from build123d import *

# Parameters (mm, degrees)
F0_W          = 457.2
F0_H          = 368.3
F1_DEPTH      = 6.35
F2_W          = 19.05
F2_H          = 330.2
F2_W_2        = 177.8
F2_H_2        = 19.05
F3_DEPTH      = 63.5
F4_W          = 203.2
F4_H          = 38.1
F4_W_2        = 374.65
F5_DEPTH      = 19.05
F8_DEPTH      = 125.9670187868
F8_DEPTH_BACK = 65.6385295619


# Not quite as in the source:
# - a feature names something its author has since deleted; it is built from what else it names


with BuildPart() as f1:
    # F0 (on Top) → F1 (new body)
    with BuildSketch(Plane.XY):
        with Locations((228.6, 184.15)):
            Rectangle(F0_W, F0_H)
    extrude(amount=F1_DEPTH)

    # F2 (on face) → F3 (join)
    with BuildSketch(Plane.XY.offset(6.35)):
        with Locations((9.525, 184.15)):
            Rectangle(F2_W, F2_H)
        Polygon((0, 368.3), (0, 349.25), (19.05, 349.25), (457.2, 349.25), (457.2, 368.3), align=None)
        Polygon((0, 19.05), (0, 0), (457.2, 0), (457.2, 19.05), (19.05, 19.05), align=None)
        with Locations((546.1, 9.525)):
            Rectangle(F2_W_2, F2_H_2)
        with Locations((546.1, 358.775)):
            Rectangle(F2_W_2, F2_H_2)
    extrude(amount=F3_DEPTH)

    # F4 (on face) → F5 (join)
    with BuildSketch(Plane.XY.offset(69.85)):
        with Locations((120.65, 120.65)):
            Rectangle(F4_W, F4_H)
        Polygon((222.25, 101.6), (222.25, 19.05), (260.35, 19.05), (260.35, 196.85), (260.35, 234.95), (260.35, 349.25), (222.25, 349.25), (222.25, 234.95), (222.25, 196.85), (222.25, 139.7), align=None)
        with Locations((120.65, 215.9)):
            Rectangle(F4_W, F4_H)
        with Locations((447.675, 215.9)):
            Rectangle(F4_W_2, F4_H)
    extrude(amount=-F5_DEPTH)

    # F7 (on face) → F8 (cut, two sides)
    with BuildSketch(Plane(origin=(0, 22.4493572683, 61.6791021759), x_dir=(1, 0, 0), z_dir=(0, -0.3420201433, -0.9396926208))) as f8_sk:
        Polygon((643.6106, 282.7225558054), (513.744137013, -453.7867547107), (643.6106, -453.7867547107), align=None)
    extrude(amount=-F8_DEPTH, mode=Mode.SUBTRACT)
    extrude(f8_sk.sketch, amount=F8_DEPTH_BACK, mode=Mode.SUBTRACT)


solid = f1.part
The model under review builds one solid part; all positions refer to its coordinate system, in mm. A direction names the side the tool comes from. Coordinates: 2 decimals unless noted, no trailing zeros. Write each loop counter-clockwise with the first axis right and the second up, starting at its lowest first coordinate (ties: lowest second). Pieces come first, ordered by that corner, then holes. Notation, with made-up numbers: (14, 57) - (73, 57) arc R23 ccw to (73, 86) - close; hole circle Ø7 at (65.5, 21.25). An arc over 180 degrees is marked (long way). Answer as a JSON object with one key per item and string values. Group by question number.
1. Mouldability with a two-part tool opening along Z and no side actions: class faces 1 (the face through (231, 199, 69.85)), 2 (the face through (0, 187, 34)), 3 (the face through (235, 186, 6.35)) as pulls with the +Z half, pulls with the -Z half, needs draft (parallel to the pull), parting line crosses it, or undercut.
2. Clearance check with flat-ended pins moving along their axes: pin 1 Ø4 at (x, y) = (531, 215.5) entering from -Z; pin 2 Ø4 at (y, z) = (190.5, 30) entering from +X; pin 3 Ø9.5 at (y, z) = (100, 59) entering from +X. State where each tip first meets the part, or that it passes through.
3. Add section C-C (x = 280). Give the boundary of the cut face in (y, z), plus the area to 3 significant figures.
4. Machinability: for faces 4 (the face through (496, 359, 6.35)), 5 (the face through (260.35, 107, 60)), 6 (the face through (119, 139.7, 60)), which of the approach directions +Z, -Z, +X, -X, +Y, -Y give a long, thin tool a straight path to every point of the face, cutting with its end or side? Answer none if there is none.
5. Add section B-B (y = 243). Give the boundary of the cut face in (x, z), plus the area to 3 significant figures.
6. Add section A-A (x = 74). Give the boundary of the cut face in (y, z).
7. Add section D-D (y = 117.5). Give the boundary of the cut face in (x, z).
8. To check wall thickness, follow probe 1 along Y at (x, z) = (424.5, 61.5); probe 2 along Y at (x, z) = (388, 37). State the ranges of each line that lie inside material, in increasing order.
Findings:
{
 "1": {"face 1": "pulls with the +Z half", "face 2": "needs draft", "face 3": "undercut"},
 "2": {"pin 1": "z = 50.8", "pin 2": "x = 19.05", "pin 3": "x = 260.35"},
 "3": {"outline": "(0, 0) - (368.3, 0) - (368.3, 69.85) - (349.25, 69.85) - (349.25, 6.35) - (19.05, 6.35) - (19.05, 69.85) - (0, 69.85) - close; (196.85, 50.8) - (234.95, 50.8) - (234.95, 69.85) - (196.85, 69.85) - close", "area": "5,480 mm²"},
 "4": {"face 4": "-Z, +X, +Y, -Y", "face 5": "+Z, +X", "face 6": "+Z"},
 "5": {"outline": "(0, 0) - (457.2, 0) - (457.2, 6.35) - (19.05, 6.35) - (19.05, 69.85) - (0, 69.85) - close; (222.25, 50.8) - (260.35, 50.8) - (260.35, 69.85) - (222.25, 69.85) - close", "area": "4,840 mm²"},
 "6": {"outline": "(0, 0) - (368.3, 0) - (368.3, 69.85) - (349.25, 69.85) - (349.25, 6.35) - (19.05, 6.35) - (19.05, 69.85) - (0, 69.85) - close; (101.6, 50.8) - (139.7, 50.8) - (139.7, 69.85) - (101.6, 69.85) - close; (196.85, 50.8) - (234.95, 50.8) - (234.95, 69.85) - (196.85, 69.85) - close"},
 "7": {"outline": "(0, 0) - (457.2, 0) - (457.2, 6.35) - (19.05, 6.35) - (19.05, 50.8) - (260.35, 50.8) - (260.35, 69.85) - (0, 69.85) - close"},
 "8": {"probe 1": "0 to 19.05, 196.85 to 234.95, 349.25 to 368.3", "probe 2": "0 to 19.05, 349.25 to 368.3"}
}
